Part model, mm, in its own coordinate system. A direction names the side the tool comes from. Give positions to 0.01 mm unless a question says otherwise; leave off trailing zeros. Order: outer loops, then holes, each group sorted by start corner. A loop starts at its lowest first (then second) coordinate and runs counter-clockwise, first axis right, second up. Notation, with made-up numbers: M -29,-21 L -15,-21 A7 ccw -15,-13 Z; hole C 36,73 d10. An arc over 180 degrees is marked long. Answer as a JSON object with one key per item and string values.
from build123d import *

# Parameters (mm, degrees)
SKETCH1_R             = 42
SKETCH1_R_2           = 25
EXTRUDE1_DEPTH        = 50
SKETCH3_R             = 29
EXTRUDE3_DEPTH        = 15
EXTRUDE4_START        = -20
SKETCH4_R             = 29
EXTRUDE4_DEPTH        = 20
SKETCH5_R             = 31
EXTRUDE5_DEPTH        = 9
M4_TAPPED_HOLE1_D     = 3.3
M4_TAPPED_HOLE1_DEPTH = 10.1
M4_TAPPED_HOLE1_TIP   = 0.991420021


with BuildPart() as part:
    # Sketch1 → Extrude1 (new body)
    with BuildSketch(Plane(origin=(0, 0, 0), x_dir=(1, 0, 0), z_dir=(0, 1, 0))):
        with Locations(Location((0, 0, 0), (0, 0, 270))):
            Circle(SKETCH1_R)
        with Locations(Location((0, 0, 0), (0, 0, 270))):
            Circle(SKETCH1_R_2, mode=Mode.SUBTRACT)
    extrude(amount=EXTRUDE1_DEPTH)

    # Sketch3 → Extrude3 (cut)
    with BuildSketch(Plane(origin=(0, 50, 0), x_dir=(1, 0, 0), z_dir=(0, 1, 0))):
        with Locations(Location((0, 0, 0), (0, 0, 270))):
            Circle(SKETCH3_R)
    extrude(amount=-EXTRUDE3_DEPTH, mode=Mode.SUBTRACT)

    # Sketch4 → Extrude4 (cut)
    with BuildSketch(Plane.XZ.offset(EXTRUDE4_START)):
        with Locations(Location((0, 0, 0), (0, 0, 90))):
            Circle(SKETCH4_R)
    extrude(amount=EXTRUDE4_DEPTH, mode=Mode.SUBTRACT)

    # Sketch5 → Extrude5 (cut)
    with BuildSketch(Plane.XZ):
        with Locations(Location((0, 0, 0), (0, 0, 270))):
            Circle(SKETCH5_R)
    extrude(amount=-EXTRUDE5_DEPTH, mode=Mode.SUBTRACT)

    # M4 Tapped Hole1
    with Locations(Plane(origin=(-24, 0, 24), x_dir=(0, 0, -1), z_dir=(0, -1, 0))):
        with Locations((0, 0), (0, 48), (48, 0), (48, 48)):
            Hole(M4_TAPPED_HOLE1_D / 2, depth=M4_TAPPED_HOLE1_DEPTH)
            with Locations((0, 0, -(M4_TAPPED_HOLE1_DEPTH + M4_TAPPED_HOLE1_TIP / 2))):  # 118° drill point
                Cone(0, M4_TAPPED_HOLE1_D / 2, M4_TAPPED_HOLE1_TIP, mode=Mode.SUBTRACT)


solid = part.part
1. Cut at C-C on y = 43. Give the cut face in (x, z).
Worked answers:
{"outline": "C 0,0 d84; hole C 0,0 d58"}
2. Cut at A-A on z = 0. Give the cut face in (x, y).
Worked answers:
{"outline": "M -42,0 L -31,0 L -31,9 L -29,9 L -29,20 L -25,20 L -25,35 L -29,35 L -29,50 L -42,50 Z; M 25,20 L 29,20 L 29,9 L 31,9 L 31,0 L 42,0 L 42,50 L 29,50 L 29,35 L 25,35 Z"}
3. Which spindle directions (+Z, -Z, +X, -X, +Y, -Y) get a long thin tool onto all of the face, cutting with end or side? Do faces 4 (the cylindrical face through (7.509, 27.395, 23.846)), 5 (the cylindrical face through (30.736, 4.437, 4.036)), 6 (the cylindrical face through (-11.107, 42.605, 26.789)). Say none if no direction does.
Worked answers:
{"face 4": "+Y, -Y", "face 5": "-Y", "face 6": "+Y"}
4. Pin check, flat tips, straight feed: P1, Ø1, axis at y = 28.5, z = -5.5, coming from the -X side; P2, Ø5, axis at x = -14, y = 24, coming from the +Z side; P3, Ø4, axis at x = -17, y = 18.5, coming from the +Z side; P4, Ø5.5, axis at x = 24, z = 24, coming from the -Y side. Stop position of each tip, or through.
Worked answers:
{"P1": "stops at x = -41.7", "P2": "stops at z = 40.39", "P3": "stops at z = 39.23", "P4": "stops at y = 0"}
5. Two-plate mould, pull along Z, no slides. Class faces 1 (the flat face through (-27.412, 50, -9.921)), 2 (the flat face through (-21, 9, -21)), 3 (the cylindrical face through (12.62, 24.65, 40.06)): +Z half, -Z half, draft (parallel to the pull), parting line (faces both ways), or undercut.
Worked answers:
{"face 1": "draft", "face 2": "undercut", "face 3": "parting line"}
6. Probe line 1 along X through (y, z) = (27, 0); line 2 along Z through (x, y) = (24, 5); line 3 along X through (y, z) = (11.5, 0). List the from-to ranges inside material, lowest first.
Worked answers:
{"line 1": "x = -42 to -25, 25 to 42", "line 2": "z = -34.47 to -25.65, -22.35 to -19.62, 19.62 to 22.35, 25.65 to 34.47", "line 3": "x = -42 to -29, 29 to 42"}
7. Cut at D-D on z = -27.5. Give the cut face in (x, y), plus the area to 3 significant figures.
Worked answers:
{"outline": "M -31.75,0 L -14.31,0 L -14.31,9 L -9.21,9 L -9.21,20 L 9.21,20 L 9.21,9 L 14.31,9 L 14.31,0 L 31.75,0 L 31.75,50 L 9.21,50 L 9.21,35 L -9.21,35 L -9.21,50 L -31.75,50 Z", "area": "2,440 mm^2"}
8. Cut at B-B on x = 0. Give the cut face in (y, z).
Worked answers:
{"outline": "M 0,-42 L 50,-42 L 50,-29 L 35,-29 L 35,-25 L 20,-25 L 20,-29 L 9,-29 L 9,-31 L 0,-31 Z; M 0,31 L 9,31 L 9,29 L 20,29 L 20,25 L 35,25 L 35,29 L 50,29 L 50,42 L 0,42 Z"}
